Autodesk Inventor part; units mm, degrees
ref_plane "YZ Plane" through (0, 0, 0) normal (1, 0, 0) x (0, 1, 0)
ref_plane "XZ Plane" through (0, 0, 0) normal (0, 1, 0) x (-1, 0, 0)
ref_plane "XY Plane" through (0, 0, 0) normal (0, 0, 1) x (1, 0, 0)
sketch "Sketch1" plane through (0, 0, 0) normal (1, 0, 0) x (0, 1, 0)
  circle A0 centre (0, 0) radius 18
  dimension "d0" = 36
extrude "Extrusion1" add sketch "Sketch1" along normal mid plane 25
sketch "Sketch2" plane through (0, 0, 0) normal (1, 0, 0) x (0, 1, 0)
  circle A0 centre (0, 0) radius 25
  dimension "d3" = 50
extrude "Extrusion2" add sketch "Sketch2" along normal mid plane 6.35
sketch "Sketch3" plane through (12.5, 0, 0) normal (1, 0, 0) x (0, 0, -1)
  line L0 (-1.5, -1.5) -> (1.5, -1.5)
  line L1 (1.5, -1.5) -> (1.5, 1.5)
  line L2 (1.5, 1.5) -> (-1.5, 1.5)
  line L3 (-1.5, 1.5) -> (-1.5, -1.5)
  line L4 (-1.5, -1.5) -> (1.5, 1.5) construction
  line L5 (1.5, -1.5) -> (-1.5, 1.5) construction
  point P0 (0, 0)
  dimension "d6" = 3
  dimension "d7" = 3
extrude "Extrusion3" cut sketch "Sketch3" against normal blind 25.4
properties part number "Sprocket"
The model under review builds one solid part; all positions refer to its coordinate system, in mm. A direction names the side the tool comes from. Round coordinates to 2 decimals unless told otherwise and drop trailing zeros. Write each loop counter-clockwise with the first axis right and the second up, starting at its lowest first coordinate (ties: lowest second). Pieces come first, ordered by that corner, then holes. Notation, with made-up numbers: (67.25, 13.25) - (85.25, 13.25) arc R27 ccw to (85.25, 39.25) - close; hole circle Ø10 at (62, 65). An arc over 180 degrees is marked (long way). Answer as CSV lines item,"result". Start each with the question number.
(1) We need section D-D on y = -16.5. State the section outline as (x, z) points (3 decimals).
(2) We need section C-C on x = -0.5. State the section outline as (y, z) points, plus the area to 3 significant figures.
(3) To check wall thickness, follow line 1 (Z direction, x = -11.25, y = 0.5); line 2 (X direction, y = -16, z = 11.5) (3 decimals); line 3 (Z direction, x = -2.75, y = -17). State the ranges of each line that lie inside material, in increasing order.
(4) Draft analysis for pull direction Y (two halves, no side actions). For faces 5 (the flat face through (12.5, 0, -4)), 6 (the cylindrical face through (-0.044, 23.846, -7.509)), 7 (the flat face through (0, -1.5, 0)), state which applies: pulls with the +Y half, pulls with the -Y half, needs draft (parallel to the pull), parting line crosses it, or undercut.
(5) For pin 1 Ø3.5 at (x, y) = (-2, -0.5) entering from -Z; pin 2 Ø4 at (x, z) = (7.5, -6.5) entering from -Y; pin 3 Ø2 at (x, z) = (2.5, -15) entering from +Y; pin 4 Ø10 at (x, z) = (-6, -2.5) entering from +Y, all flat-tipped, find the tip position at first contact; note any pin that passes through.
(6) We need section A-A on z = 0. State the section outline as (x, y) points (3 decimals).
(7) For faces 1 (the flat face through (3.175, 11, -16)), 2 (the flat face through (0, 0, 1.5)), 3 (the flat face through (-3.175, 11, -16)), 4 (the flat face through (-12.5, 0, -4)), list the 3-axis set-ups (+Z, -Z, +X, -X, +Y, -Y) from which the entire face can be reached by the end or side of a thin tool; tool diameter is ignored.
Worked answers:
1,outline,"(-12.5, -7.194) - (-3.175, -7.194) - (-3.175, -18.782) - (3.175, -18.782) - (3.175, -7.194) - (12.5, -7.194) - (12.5, 7.194) - (3.175, 7.194) - (3.175, 18.782) - (-3.175, 18.782) - (-3.175, 7.194) - (-12.5, 7.194) - close"
2,outline,"circle Ø50 at (0, 0); hole (-1.5, -1.5) - (1.5, -1.5) - (1.5, 1.5) - (-1.5, 1.5) - close"
2,area,"1,950 mm²"
3,line 1,"-17.99 to -1.5, 1.5 to 17.99"
3,line 2,"-3.175 to 3.175"
3,line 3,"-18.33 to 18.33"
4,face 5,"needs draft"
4,face 6,"parting line crosses it"
4,face 7,"undercut"
5,pin 1,"z = -25"
5,pin 2,"y = -17.43"
5,pin 3,"y = 20.71"
5,pin 4,"y = 25"
6,outline,"(-12.5, -18) - (-3.175, -18) - (-3.175, -25) - (3.175, -25) - (3.175, -18) - (12.5, -18) - (12.5, -1.5) - (-12.5, -1.5) - close; (-12.5, 1.5) - (12.5, 1.5) - (12.5, 18) - (3.175, 18) - (3.175, 25) - (-3.175, 25) - (-3.175, 18) - (-12.5, 18) - close"
7,face 1,"+X"
7,face 2,"+X, -X"
7,face 3,"-X"
7,face 4,"+Z, -Z, -X, +Y, -Y"
